Build history of the part. All positions in model axes, mm. Face numbers are marked on the shaded views. A direction names the side the tool comes from. Coordinates: 2 decimals unless noted, no trailing zeros. Write each loop counter-clockwise with the first axis right and the second up, starting at its lowest first coordinate (ties: lowest second). Pieces come first, ordered by that corner, then holes. Notation, with made-up numbers: M -40,-0.5 L -4,-0.5 A11 ccw -4,15.5 Z; hole C -4,-21.5 d2. An arc over 180 degrees is marked long. Use CSV: the item, a comma, the result in double quotes. Start each with the question number.
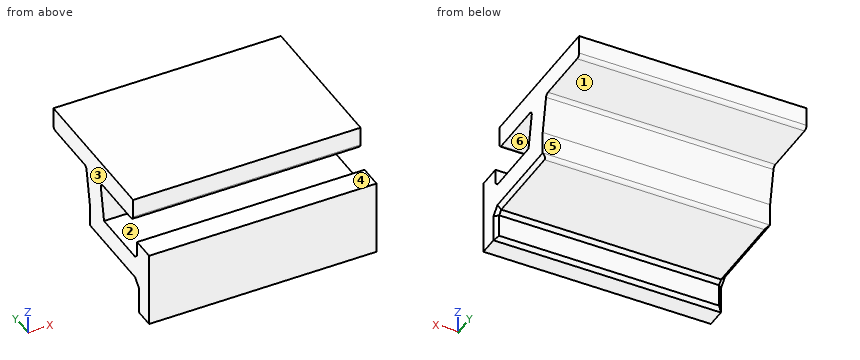
```python
from build123d import *

# Parameters (mm, degrees)
BOSS_EXTRUDE1_DEPTH = 30
CHAMFER1_SIZE       = 0.5
FILLET1_R           = 0.5


with BuildPart() as part:
    # Sketch1 → Boss-Extrude1 (new body)
    with BuildSketch(Plane(origin=(0, 0, 0), x_dir=(0, 0, -1), z_dir=(1, 0, 0))):
        Polygon((-5, 0), (-5, 3), (-2.5, 3), (-2.5, 11.309733412), (-7.5, 12.221162959), (-7.5, 4), (-10.5, 4), (-10.5, 24), (-7.5, 24), (-7.5, 15.778837041), (-2.5, 14.867407493), (1, 14.867407493), (1, 3), (5, 3), (5, 0), align=None)
    extrude(amount=BOSS_EXTRUDE1_DEPTH)

    # Chamfer1
    chamfer1_edges = [part.edges().sort_by_distance(p)[0] for p in [
        (15, 3, 2.5),
        (0, 3, -3),
        (30, 8.933703747, -1),
        (0, 8.933703747, -1),
        (15, 3, -5),
        (30, 3, -3),
        (15, 3, -1),
    ]]
    chamfer(chamfer1_edges, length=CHAMFER1_SIZE)

    # Fillet1
    fillet1_edges = [part.edges().sort_by_distance(p)[0] for p in [
        (15, 4, 7.5),
        (15, 24, 7.5),
        (15, 12.221162959, 7.5),
        (15, 15.778837041, 7.5),
        (15, 14.867407493, -1),
    ]]
    fillet(fillet1_edges, radius=FILLET1_R)


solid = part.part
```
1. Pull direction Z, two halves, no side cores. Call the marked faces 4, 5 and 6: pulls with the +Z half, pulls with the -Z half, needs draft (parallel to the pull), parting line crosses it, or undercut.
2. Slice it at C-C (x = 9.25). List the corners of the cut face in (y, z).
3. Drill centre lines: line 1 along Z through (x, y) = (19, 6.5); line 2 along Y through (x, z) = (7.75, 0); line 3 along Y through (x, z) = (23.5, 4.75). Where is each one in solid material? Low to high. Write a range as from..to.
4. Slice it at B-B (z = -3.25). List the corners of the cut face in (x, y), and give its area (4 significant figures).
5. Slice it at D-D (y = 13.5). List the corners of the cut face in (x, z).
6. 3-axis set-ups, long thin cutter, end or side, ignore diameter. For the marked faces 1, 2 and 3: which of +Z, -Z, +X, -X, +Y, -Y reach the whole face in a straight line?
7. Flat gauge pins, fed straight in: pin 1 (3.5 mm diameter, centred on x = 12, y = 1.5, fed in from +Z); pin 2 (5.5 mm diameter, centred on x = 22, y = 9, fed in from -Z); pin 3 (2.5 mm diameter, centred on x = 8.5, z = -3, fed in from +Y); pin 4 (1 mm diameter, centred on y = 7.5, z = -2.5, fed in from -X). Where does each tip first touch, or does it go through?
8. Slice it at A-A (y = 6.25). List the corners of the cut face in (x, z), and give its area (3 significant figures).
Established:
1,face 4,"pulls with the +Z half"
1,face 5,"needs draft"
1,face 6,"undercut"
2,outline,"M 0,-5 L 2.5,-5 L 3,-4.5 L 3,-1.5 L 3.5,-1 L 14.37,-1 A0.5 ccw 14.87,-0.5 L 14.87,2.5 L 15.7,7.09 A0.5 cw 16.2,7.5 L 23.5,7.5 A0.5 ccw 24,8 L 24,10.5 L 4,10.5 L 4,8 A0.5 ccw 4.5,7.5 L 11.62,7.5 A0.5 cw 12.11,6.91 L 11.31,2.5 L 3.5,2.5 L 3,3 L 3,5 L 0,5 Z"
3,line 1,"z = -1..2.5, 7.5..10.5"
3,line 2,"y = 0..14.87"
3,line 3,"y = 0..3, 11.72..15.28"
4,outline,"M 0,0 L 30,0 L 30,2.5 L 29.5,3 L 0.5,3 L 0,2.5 Z"
4,area,"89.75 mm2"
5,outline,"M 0,-0.5 L 0.5,-1 L 29.5,-1 L 30,-0.5 L 30,10.5 L 0,10.5 Z"
6,face 1,"-Z, +X, -X, +Y"
6,face 2,"+X, -X"
6,face 3,"+Z, -Z, -X, +Y, -Y"
7,pin 1,"stops at z = 5"
7,pin 2,"stops at z = -1"
7,pin 3,"stops at y = 3"
7,pin 4,"passes through"
8,outline,"M 0,-0.5 L 0.5,-1 L 29.5,-1 L 30,-0.5 L 30,2.5 L 0,2.5 Z; M 0,7.5 L 30,7.5 L 30,10.5 L 0,10.5 Z"
8,area,"195 mm2"
